Geometry check sheet. Reference: drawing and pictorial views, mm from the part's lowest x, y, z. Round coordinates to 2 decimals unless told otherwise and drop trailing zeros. Write each loop counter-clockwise with the first axis right and the second up, starting at its lowest first coordinate (ties: lowest second). Pieces come first, ordered by that corner, then holes. Notation, with made-up numbers: M -15,-25 L 6,-25 A22 ccw 6,-5 Z; hole C -2,-2.5 d1. An arc over 180 degrees is marked long. Answer in a Markdown table with one row per item.
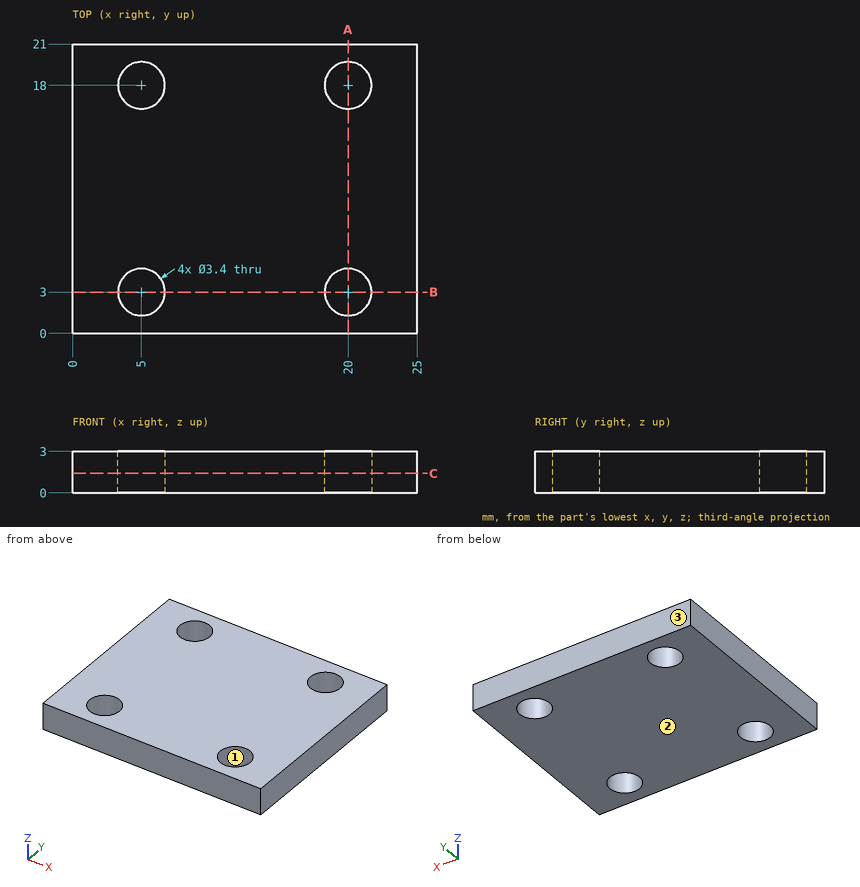
1. Go/stop test with a flat-tipped pin: pin 1 (2.5 mm diameter, centred on x = 20, y = 18, fed in from +Z). Record where the tip stops, or that it passes through.
Found:
| item | result |
|---|---|
| pin 1 | passes through |
2. Section check C-C, the plane z = 1.4. Record the cut outline in (x, y), and give its area (3 significant figures).
Found:
| item | result |
|---|---|
| outline | M 0,0 L 25,0 L 25,21 L 0,21 Z; hole C 5,3 d3.4; hole C 5,18 d3.4; hole C 20,3 d3.4; hole C 20,18 d3.4 |
| area | 489 mm2 |
3. Scan lines: L1, parallel to Y at x = 20, z = 1.4; L2, parallel to Y at x = 4.5, z = 2.7; L3, parallel to X at y = 18.5, z = 1.9. Record each from-to range of solid material in increasing order.
Found:
| item | result |
|---|---|
| L1 | y = 0 to 1.3, 4.7 to 16.3, 19.7 to 21 |
| L2 | y = 0 to 1.38, 4.62 to 16.38, 19.62 to 21 |
| L3 | x = 0 to 3.38, 6.62 to 18.38, 21.62 to 25 |
4. Section check A-A, the plane x = 20. Record the cut outline in (y, z).
Found:
| item | result |
|---|---|
| outline | M 0,0 L 1.3,0 L 1.3,3 L 0,3 Z; M 4.7,0 L 16.3,0 L 16.3,3 L 4.7,3 Z; M 19.7,0 L 21,0 L 21,3 L 19.7,3 Z |
5. Draft check along Y on the marked faces 1, 2 and 3. Enter one of: +Y half, -Y half, draft (parallel to the pull), parting line (faces both ways), or undercut.
Found:
| item | result |
|---|---|
| face 1 | undercut |
| face 2 | draft |
| face 3 | +Y half |
6. Section check B-B, the plane y = 3. Record the cut outline in (x, z).
Found:
| item | result |
|---|---|
| outline | M 0,0 L 3.3,0 L 3.3,3 L 0,3 Z; M 6.7,0 L 18.3,0 L 18.3,3 L 6.7,3 Z; M 21.7,0 L 25,0 L 25,3 L 21.7,3 Z |
